Source: CAD feature listing. Evaluate the final solid. Frame: model axes, mm. A direction names the side the tool comes from. Coordinates: 2 decimals unless noted, no trailing zeros. Order: outer loops, then holes, each group sorted by start corner. A loop starts at its lowest first (then second) coordinate and runs counter-clockwise, first axis right, second up. Notation, with made-up numbers: (-0.5, 77) - (13.5, 77) arc R8 ccw to (13.5, 89) - close; hole circle Ø9 at (-5.5, 78). An arc over 180 degrees is marked (long way). One line per question, with ' | ' between items.
from build123d import *

# Parameters (mm, degrees)
F0_W     = 35
F0_H     = 25
F1_DEPTH = 3
F2_W     = 3
F2_H     = 25
F3_DEPTH = 40
F4_R     = 12.49999
F5_R     = 12.49999
F6_R     = 16
F7_DEPTH = 21
F8_R     = 14.5
F9_DEPTH = 18


# Not quite as in the source:
# - a fillet or chamfer is up to 0.001 mm smaller than in the source, because OpenCascade refuses the exact size


with BuildPart() as f1:
    # F0 (on Top) → F1 (new body)
    with BuildSketch(Plane.XY):
        Rectangle(F0_W, F0_H)
    extrude(amount=F1_DEPTH)

    # F2 (on Top) → F3 (join)
    with BuildSketch(Plane.XY):
        with Locations((16, 0)):
            Rectangle(F2_W, F2_H)
    extrude(amount=F3_DEPTH)

    # F4 (radius 12.5 in the source; OpenCascade refuses exactly that, so slightly less here)
    f4_edges = [f1.edges().sort_by_distance(p)[0] for p in [
        (-17.5, 12.5, 1.5),
        (-17.5, -12.5, 1.5),
    ]]
    fillet(f4_edges, radius=F4_R)

    # F5 (radius 12.5 in the source; OpenCascade refuses exactly that, so slightly less here)
    f5_edges = [f1.edges().sort_by_distance(p)[0] for p in [
        (16, 12.5, 40),
        (16, -12.5, 40),
    ]]
    fillet(f5_edges, radius=F5_R)

    # F6 (on face) → F7 (join)
    with BuildSketch(Plane(origin=(14.5, 0, 0), x_dir=(0, -1, 0), z_dir=(-1, 0, 0))):
        with Locations((0, 30)):
            Circle(F6_R)
    extrude(amount=-F7_DEPTH)

    # F8 (on face) → F9 (cut)
    with BuildSketch(Plane(origin=(14.5, 0, 0), x_dir=(0, -1, 0), z_dir=(-1, 0, 0))):
        with Locations((0, 30)):
            Circle(F8_R)
    extrude(amount=-F9_DEPTH, mode=Mode.SUBTRACT)


solid = f1.part
(1) Cut plane A-A (z = 30). Return the cut outline in (x, y).
Taken from the geometry:
outline: (14.5, -16) - (35.5, -16) - (35.5, 16) - (14.5, 16) - (14.5, 14.5) - (32.5, 14.5) - (32.5, -14.5) - (14.5, -14.5) - close
(2) Cut plane D-D (x = 11). Return the cut outline in (y, z).
Taken from the geometry:
outline: (-12.5, 0) - (12.5, 0) - (12.5, 3) - (-12.5, 3) - close
(3) Cut plane C-C (y = 11). Return the cut outline in (x, z), and give its area (3 significant figures).
Taken from the geometry:
outline: (-10.94, 0) - (17.5, 0) - (17.5, 18.38) - (35.5, 18.38) - (35.5, 41.62) - (14.5, 41.62) - (14.5, 39.45) - (32.5, 39.45) - (32.5, 20.55) - (14.5, 20.55) - (14.5, 3) - (-10.94, 3) - close | area: 279 mm²
(4) Cut plane B-B (x = 23). Return the cut outline in (y, z).
Taken from the geometry:
outline: circle Ø32 at (0, 30); hole circle Ø29 at (0, 30)
(5) Material intervals for L1, parallel to Z at x = 20, y = 0; L2, parallel to Z at x = -13, y = -8.5; L3, parallel to X at y = -11, z = 30.5, sorted ascending. Write a range as from..to.
Taken from the geometry:
L1: z = 14..15.5, 44.5..46 | L2: z = 0..3 | L3: x = 32.5..35.5
(6) Pin query (flat end, axial travel): P1, Ø8, axis at x = 2, y = -0.5, coming from the +Z side; P2, Ø22, axis at x = 9.5, z = 9, coming from the -Y side; P3, Ø5, axis at y = -6.5, z = 33, coming from the -X side. Return the tip coordinate at first contact, or that it passes through.
Taken from the geometry:
P1: stops at z = 3 | P2: stops at y = -12.5 | P3: stops at x = 32.5
(7) Set-up query: faces 5 (the flat face through (11.2, -12.5, 2.5)), 6 (the cylindrical face through (-13.741, 8.935, 1.521)), 7 (the cylindrical face through (24.853, 2.083, 45.864)), 8 (the flat face through (14.5, 1, 15)), 9 (the cylindrical face through (-13.741, -8.935, 1.521)). Return all of +Z, -Z, +X, -X, +Y, -Y with unobstructed straight access to the full face (end or side cutting, diameter ignored); none if empty.
Taken from the geometry:
face 5: -Z, +X, -X, -Y | face 6: +Z, -Z, -X, +Y | face 7: +X | face 8: +Z, -X, +Y, -Y | face 9: +Z, -Z, -X, -Y
(8) Pull-direction query (Y, two-part tool) for faces 1 (the flat face through (11.2, 12.5, 2.5)), 2 (the flat face through (35.5, 0, 30)), 3 (the cylindrical face through (23.374, 1.888, 44.377)), 4 (the flat face through (32.5, 0, 30)); classes: pulls with the +Y half, pulls with the -Y half, needs draft (parallel to the pull), parting line crosses it, or undercut.
Taken from the geometry:
face 1: pulls with the +Y half | face 2: needs draft | face 3: undercut | face 4: undercut
